from build123d import *

# Parameters (mm, degrees)
F2_R     = 27.25
F3_DEPTH = 45.001


with BuildPart() as f1:
    # F0 (on Front) → F1 (revolve)
    with BuildSketch(Plane.XZ):
        Polygon((-51, 0), (0, 0), (0, 45), (-31.2, 45), (-31.2, 37), (-47, 3), (-53, 3), align=None)
    revolve(axis=Axis((0, 0, 22.5), (0, 0, 1)))

    # F2 (on face) → F3 (cut, through all)
    with BuildSketch(Plane.XY.offset(45)):
        Circle(F2_R)
    extrude(amount=-F3_DEPTH, mode=Mode.SUBTRACT)


solid = f1.part
The listing builds one solid part. Answer for the finished solid, in the listing's coordinates (mm). A direction names the side the tool comes from. Coordinates: 2 decimals unless noted, no trailing zeros. Order: outer loops, then holes, each group sorted by start corner. A loop starts at its lowest first (then second) coordinate and runs counter-clockwise, first axis right, second up. Notation, with made-up numbers: (-34.5, -17.5) -> (-11.5, -17.5) arc R6 cw to (-11.5, -8.5) -> close; hole circle Ø5 at (-39, 59). An arc over 180 degrees is marked (long way). Answer in a Markdown table with one row per item. Add a question column.
Item 1: Each of these flat-tipped pins is pushed along its axis until it touches: P1, Ø1, axis at y = -28, z = 36.5, coming from the +X side; P2, Ø2, axis at y = 27, z = 39.5, coming from the -X side; P3, Ø4, axis at x = -22.5, z = 8, coming from the -Y side. Where does it stop, or does it pass through?
Item 2: Find section A-A (y = 0). Write down the section's boundary in (x, z).
Item 3: Find section C-C (z = 18.5). Write down the section's boundary in (x, y).
Item 4: Find section D-D (z = 10). Write down the section's boundary in (x, y), then the cut area to 3 significant figures.
Item 5: Determine the mould class of faces 3 (the face through (0, 28, 45)), 4 (the face through (-21.625, -16.581, 22.815)), 5 (the face through (22.996, -21.086, 40.944)) for opening direction Y: +Y half, -Y half, draft (parallel to the pull), parting line (faces both ways), or undercut.
Item 6: Find the intervals of material crossed by L1, parallel to X at y = -4, z = 39; L2, parallel to Y at x = 0, z = 28.5; L3, parallel to Y at x = 6, z = 38.5, in increasing order. Write a range as from..to.
Item 7: Which of the six approach directions +Z, -Z, +X, -X, +Y, -Y give full straight-line access (tool end or side, diameter ignored) to faces 1 (the face through (-22, 22, 0)), 2 (the face through (-4, 47, 3))?
Result set:
| question | item | result |
|---|---|---|
| 1 | P1 | stops at x = 15.34 |
| 1 | P2 | stops at x = -17.25 |
| 1 | P3 | stops at y = -40.13 |
| 2 | outline | (-53, 3) -> (-51, 0) -> (-27.25, 0) -> (-27.25, 45) -> (-31.2, 45) -> (-31.2, 37) -> (-47, 3) -> close; (27.25, 0) -> (51, 0) -> (53, 3) -> (47, 3) -> (31.2, 37) -> (31.2, 45) -> (27.25, 45) -> close |
| 3 | outline | circle Ø79.59 at (0, 0); hole circle Ø54.5 at (0, 0) |
| 4 | outline | circle Ø87.49 at (0, 0); hole circle Ø54.5 at (0, 0) |
| 4 | area | 3,680 mm² |
| 5 | face 3 | draft |
| 5 | face 4 | undercut |
| 5 | face 5 | parting line |
| 6 | L1 | x = -30.94..-26.95, 26.95..30.94 |
| 6 | L2 | y = -35.15..-27.25, 27.25..35.15 |
| 6 | L3 | y = -30.62..-26.58, 26.58..30.62 |
| 7 | face 1 | -Z, +X, -X, +Y, -Y |
| 7 | face 2 | +Z |
